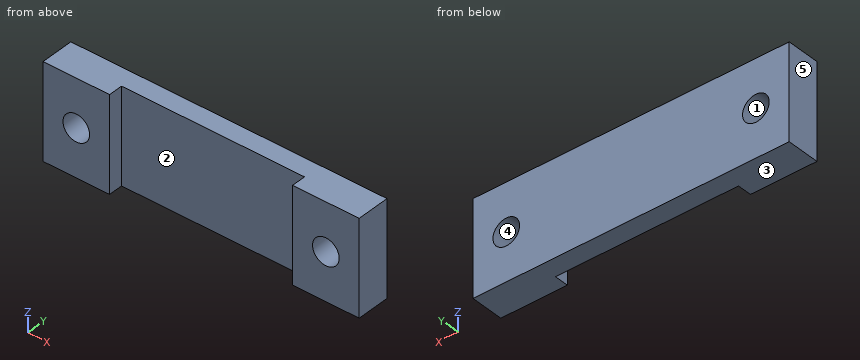
from build123d import *

# Parameters (mm, degrees)
SKETCH1_W             = 7
SKETCH1_H             = 10
SKETCH1_R             = 1.4
BOSS_EXTRUDE1_DEPTH   = 3.5
BOSS_EXTRUDE1_2_DEPTH = 3.5
SKETCH1_3_W           = 19.24
SKETCH1_3_H           = 10
BOSS_EXTRUDE2_DEPTH   = 2


with BuildPart() as part:
    # Sketch1 → Boss-Extrude1 (new body)
    with BuildSketch(Plane(origin=(0, 0, 0), x_dir=(1, 0, 0), z_dir=(0, 1, 0))):
        with Locations((-13.12, 0)):
            Rectangle(SKETCH1_W, SKETCH1_H)
        with Locations(Location((-13.12, 0, 0), (0, 0, 270))):
            Circle(SKETCH1_R, mode=Mode.SUBTRACT)
    extrude(amount=-BOSS_EXTRUDE1_DEPTH)



with BuildPart() as body_2:
    # Sketch1 → Boss-Extrude1 2 (new body)
    with BuildSketch(Plane(origin=(0, 0, 0), x_dir=(1, 0, 0), z_dir=(0, 1, 0))):
        with Locations((13.12, 0)):
            Rectangle(SKETCH1_W, SKETCH1_H)
        with Locations(Location((13.12, 0, 0), (0, 0, 270))):
            Circle(SKETCH1_R, mode=Mode.SUBTRACT)
    extrude(amount=-BOSS_EXTRUDE1_2_DEPTH)


with BuildPart() as part_1:
    add(part.part)

    add(body_2.part)  # Boss-Extrude2 merges body 2
    # Sketch1_3 → Boss-Extrude2 (add)
    with BuildSketch(Plane(origin=(0, 0, 0), x_dir=(1, 0, 0), z_dir=(0, 1, 0))):
        Rectangle(SKETCH1_3_W, SKETCH1_3_H)
    extrude(amount=-BOSS_EXTRUDE2_DEPTH)


solid = part_1.part
For this review, take the finished solid that the model builds, in its own axes (mm). Face numbers are marked on the shaded views. A direction names the side the tool comes from. Round coordinates to 2 decimals unless told otherwise and drop trailing zeros. Write each loop counter-clockwise with the first axis right and the second up, starting at its lowest first coordinate (ties: lowest second). Pieces come first, ordered by that corner, then holes. Notation, with made-up numbers: M 77.25,11 L 95.25,11 A11 cw 95.25,31 Z; hole C 66,45 d2. An arc over 180 degrees is marked long. Write item = value, one per line. Start each with the question number.
(1) For the marked faces 1 and 2, list the 3-axis set-ups (+Z, -Z, +X, -X, +Y, -Y) from which the entire face can be reached by the end or side of a thin tool; tool diameter is ignored.
(2) We need section C-C (x = -13.12). Give the boundary of the cut face in (y, z).
(3) We need section A-A (z = 0). Give the boundary of the cut face in (x, y).
(4) We need section D-D (z = -2.5). Give the boundary of the cut face in (x, y).
(5) For line 1 along X through (y, z) = (-2.7, 0); line 2 along X through (y, z) = (-0.9, 0); line 3 along Z through (x, y) = (13, -3.3), list the stretches that pass through material, from the lowest coordinate up.
(6) Clearance check with a flat-ended pin moving along its axis: pin 1 Ø5 at (x, z) = (-2, -0.5) entering from -Y. State where the tip first meets the part, or that it passes through.
(7) The part is to be moulded in two halves that separate along Z. For the marked faces 3, 4 and 5, say which applies: +Z half, -Z half, draft (parallel to the pull), parting line (faces both ways), or undercut.
(8) We need section B-B (y = -1.15). Give the boundary of the cut face in (x, z).
Results found:
q1.face_1 = +Y, -Y
q1.face_2 = +Z, -Z, -Y
q2.outline = M -3.5,-5 L 0,-5 L 0,-1.4 L -3.5,-1.4 Z; M -3.5,1.4 L 0,1.4 L 0,5 L -3.5,5 Z
q3.outline = M -16.62,-3.5 L -14.52,-3.5 L -14.52,0 L -16.62,0 Z; M -11.72,-3.5 L -9.62,-3.5 L -9.62,-2 L 9.62,-2 L 9.62,-3.5 L 11.72,-3.5 L 11.72,0 L -11.72,0 Z; M 14.52,-3.5 L 16.62,-3.5 L 16.62,0 L 14.52,0 Z
q4.outline = M -16.62,-3.5 L -9.62,-3.5 L -9.62,-2 L 9.62,-2 L 9.62,-3.5 L 16.62,-3.5 L 16.62,0 L -16.62,0 Z
q5.line_1 = -16.62 to -14.52, -11.72 to -9.62, 9.62 to 11.72, 14.52 to 16.62
q5.line_2 = -16.62 to -14.52, -11.72 to 11.72, 14.52 to 16.62
q5.line_3 = -5 to -1.39, 1.39 to 5
q6.pin_1 = -2
q7.face_3 = -Z half
q7.face_4 = undercut
q7.face_5 = draft
q8.outline = M -16.62,-5 L 16.62,-5 L 16.62,5 L -16.62,5 Z; hole C -13.12,0 d2.8; hole C 13.12,0 d2.8
